Geometry check sheet. Reference: the model listing, model coordinates, mm. A direction names the side the tool comes from. Coordinates: 2 decimals unless noted, no trailing zeros. Write each loop counter-clockwise with the first axis right and the second up, starting at its lowest first coordinate (ties: lowest second). Pieces come first, ordered by that corner, then holes. Notation, with made-up numbers: M 21,-30.5 L 47,-30.5 A22 ccw 47,-17.5 Z; hole C 80,33.5 d1. An arc over 180 degrees is marked long. Answer as a JSON object with one key per item and string values. Group by question number.
```python
from build123d import *

# Parameters (mm, degrees)
SKETCH1_W           = 12.7
SKETCH1_H           = 12.7
BOSS_EXTRUDE1_DEPTH = 190
SKETCH2_R           = 3.125
CUT_EXTRUDE1_DEPTH  = 10
CHAMFER1_SIZE       = 2


with BuildPart() as part:
    # Sketch1 → Boss-Extrude1 (new, symmetric)
    with BuildSketch(Plane.XY):
        Rectangle(SKETCH1_W, SKETCH1_H)
    extrude(amount=BOSS_EXTRUDE1_DEPTH, both=True)

    # Sketch2 → Cut-Extrude1 (cut)
    with BuildSketch(Plane.XY.offset(190)):
        Circle(SKETCH2_R)
    extrude(amount=-CUT_EXTRUDE1_DEPTH, mode=Mode.SUBTRACT)

    # Chamfer1
    chamfer1_edges = [part.edges().sort_by_distance(p)[0] for p in [
        (-6.35, 6.35, 0),
        (-6.35, -6.35, 0),
        (6.35, -6.35, 0),
        (6.35, 6.35, 0),
    ]]
    chamfer(chamfer1_edges, length=CHAMFER1_SIZE)


solid = part.part
```
1) Material ranges on probe 1 along Y at (x, z) = (0, 184.25) (3 decimals); probe 2 along Z at (x, y) = (1.75, 2); probe 3 along X at (y, z) = (-5.75, 148), recorded low to high. Write a range as [from, to].
2) Section check A-A (z = -51). Record the cut outline in (x, y), then the cut area to 3 significant figures.
3) Go/stop test with a flat-tipped pin: pin 1 Ø5 at (x, y) = (0, 0) entering from +Z. Record where the tip stops, or that it passes through.
4) Draft check along Y on faces 1 (the flat face through (0, 0, -190)), 2 (the flat face through (0, -6.35, 3)), 3 (the cylindrical face through (2.98, 0.94, 185.07)), 4 (the flat face through (0, 6.35, 3)). Enter one of: +Y half, -Y half, draft (parallel to the pull), parting line (faces both ways), or undercut.
5) Set-up check for faces 5 (the flat face through (-2, 3, 190)), 6 (the flat face through (0, 0, 180)): record each of +Z, -Z, +X, -X, +Y, -Y from which the full face is reachable in a straight line by a thin tool's end or side.
Entries:
{
 "1": {"probe 1": "[-6.35, -3.125], [3.125, 6.35]", "probe 2": "[-190, 180]", "probe 3": "[-4.95, 4.95]"},
 "2": {"outline": "M -6.35,-4.35 L -4.35,-6.35 L 4.35,-6.35 L 6.35,-4.35 L 6.35,4.35 L 4.35,6.35 L -4.35,6.35 L -6.35,4.35 Z", "area": "153 mm^2"},
 "3": {"pin 1": "z = 180"},
 "4": {"face 1": "draft", "face 2": "-Y half", "face 3": "undercut", "face 4": "+Y half"},
 "5": {"face 5": "+Z, +X, -X, +Y, -Y", "face 6": "+Z"}
}
